```python
from build123d import *

# Parameters (mm, degrees)
SKETCH_1_R          = 17.5
EXTRUDE_1_DEPTH     = 3
CUT_EXTRUDE_1_REACH = 26.93
SKETCH_2_R          = 1.25
CUT_EXTRUDE_2_REACH = 26.93
SKETCH_3_R          = 1.25
CUT_EXTRUDE_3_REACH = 26.93
SKETCH_4_R          = 7.5
CUT_EXTRUDE_4_REACH = 26.93
FILLET_1_R          = 3
SKETCH_8_R          = 3
CUT_EXTRUDE_5_DEPTH = 2


with BuildPart() as part:
    # 草图1 → 凸台-拉伸1 (new body)
    with BuildSketch(Plane.XY):
        Circle(SKETCH_1_R)
    extrude(amount=EXTRUDE_1_DEPTH)

    # 草图2 → 切除-拉伸1 (cut, up to next)
    with BuildSketch(Plane(origin=(0, 0, 0), x_dir=(-1, 0, 0), z_dir=(0, 0, -1)), mode=Mode.PRIVATE) as cut_extrude_1_sk1:
        with Locations((-8.838834765, 8.838834765)):
            Circle(SKETCH_2_R)
    cut_extrude_1_tool1 = extrude(cut_extrude_1_sk1.sketch, amount=-CUT_EXTRUDE_1_REACH, mode=Mode.PRIVATE) & part.part
    # 草图2 → 切除-拉伸1 (cut, up to next)
    with BuildSketch(Plane(origin=(0, 0, 0), x_dir=(-1, 0, 0), z_dir=(0, 0, -1)), mode=Mode.PRIVATE) as cut_extrude_1_sk2:
        with Locations((8.838834765, 8.838834765)):
            Circle(SKETCH_2_R)
    cut_extrude_1_tool2 = extrude(cut_extrude_1_sk2.sketch, amount=-CUT_EXTRUDE_1_REACH, mode=Mode.PRIVATE) & part.part
    # 草图2 → 切除-拉伸1 (cut, up to next)
    with BuildSketch(Plane(origin=(0, 0, 0), x_dir=(-1, 0, 0), z_dir=(0, 0, -1)), mode=Mode.PRIVATE) as cut_extrude_1_sk3:
        with Locations((8.838834765, -8.838834765)):
            Circle(SKETCH_2_R)
    cut_extrude_1_tool3 = extrude(cut_extrude_1_sk3.sketch, amount=-CUT_EXTRUDE_1_REACH, mode=Mode.PRIVATE) & part.part
    # 草图2 → 切除-拉伸1 (cut, up to next)
    with BuildSketch(Plane(origin=(0, 0, 0), x_dir=(-1, 0, 0), z_dir=(0, 0, -1)), mode=Mode.PRIVATE) as cut_extrude_1_sk4:
        with Locations((-8.838834765, -8.838834765)):
            Circle(SKETCH_2_R)
    cut_extrude_1_tool4 = extrude(cut_extrude_1_sk4.sketch, amount=-CUT_EXTRUDE_1_REACH, mode=Mode.PRIVATE) & part.part
    add(cut_extrude_1_tool1.solids().sort_by_distance((8.838835, 8.838835, 0))[0], mode=Mode.SUBTRACT)
    add(cut_extrude_1_tool2.solids().sort_by_distance((-8.838835, 8.838835, 0))[0], mode=Mode.SUBTRACT)
    add(cut_extrude_1_tool3.solids().sort_by_distance((-8.838835, -8.838835, 0))[0], mode=Mode.SUBTRACT)
    add(cut_extrude_1_tool4.solids().sort_by_distance((8.838835, -8.838835, 0))[0], mode=Mode.SUBTRACT)

    # 草图3 → 切除-拉伸2 (cut, up to next)
    with BuildSketch(Plane(origin=(0, 0, 0), x_dir=(-1, 0, 0), z_dir=(0, 0, -1)), mode=Mode.PRIVATE) as cut_extrude_2_sk1:
        with Locations((0, 10.606601718)):
            Circle(SKETCH_3_R)
    cut_extrude_2_tool1 = extrude(cut_extrude_2_sk1.sketch, amount=-CUT_EXTRUDE_2_REACH, mode=Mode.PRIVATE) & part.part
    # 草图3 → 切除-拉伸2 (cut, up to next)
    with BuildSketch(Plane(origin=(0, 0, 0), x_dir=(-1, 0, 0), z_dir=(0, 0, -1)), mode=Mode.PRIVATE) as cut_extrude_2_sk2:
        with Locations((-10.606601718, 0)):
            Circle(SKETCH_3_R)
    cut_extrude_2_tool2 = extrude(cut_extrude_2_sk2.sketch, amount=-CUT_EXTRUDE_2_REACH, mode=Mode.PRIVATE) & part.part
    # 草图3 → 切除-拉伸2 (cut, up to next)
    with BuildSketch(Plane(origin=(0, 0, 0), x_dir=(-1, 0, 0), z_dir=(0, 0, -1)), mode=Mode.PRIVATE) as cut_extrude_2_sk3:
        with Locations((0, -10.606601718)):
            Circle(SKETCH_3_R)
    cut_extrude_2_tool3 = extrude(cut_extrude_2_sk3.sketch, amount=-CUT_EXTRUDE_2_REACH, mode=Mode.PRIVATE) & part.part
    # 草图3 → 切除-拉伸2 (cut, up to next)
    with BuildSketch(Plane(origin=(0, 0, 0), x_dir=(-1, 0, 0), z_dir=(0, 0, -1)), mode=Mode.PRIVATE) as cut_extrude_2_sk4:
        with Locations((10.606601718, 0)):
            Circle(SKETCH_3_R)
    cut_extrude_2_tool4 = extrude(cut_extrude_2_sk4.sketch, amount=-CUT_EXTRUDE_2_REACH, mode=Mode.PRIVATE) & part.part
    add(cut_extrude_2_tool1.solids().sort_by_distance((0, 10.606602, 0))[0], mode=Mode.SUBTRACT)
    add(cut_extrude_2_tool2.solids().sort_by_distance((10.606602, 0, 0))[0], mode=Mode.SUBTRACT)
    add(cut_extrude_2_tool3.solids().sort_by_distance((0, -10.606602, 0))[0], mode=Mode.SUBTRACT)
    add(cut_extrude_2_tool4.solids().sort_by_distance((-10.606602, 0, 0))[0], mode=Mode.SUBTRACT)

    # 草图4 → 切除-拉伸3 (cut, up to next)
    with BuildSketch(Plane(origin=(0, 0, 0), x_dir=(-1, 0, 0), z_dir=(0, 0, -1)), mode=Mode.PRIVATE) as cut_extrude_3_sk1:
        Circle(SKETCH_4_R)
    cut_extrude_3_tool1 = extrude(cut_extrude_3_sk1.sketch, amount=-CUT_EXTRUDE_3_REACH, mode=Mode.PRIVATE) & part.part
    add(cut_extrude_3_tool1.solids().sort_by_distance((0, 0, 0))[0], mode=Mode.SUBTRACT)

    # 草图7 → 切除-拉伸4 (cut, up to next)
    with BuildSketch(Plane.XY.offset(3), mode=Mode.PRIVATE) as cut_extrude_4_sk1:
        with BuildLine():
            Line((-12.374368671, 12.374368671), (12.374368671, 12.374368671))
            ThreePointArc((12.374368671, 12.374368671), (0, 17.5), (-12.374368671, 12.374368671))
        make_face()
    cut_extrude_4_tool1 = extrude(cut_extrude_4_sk1.sketch, amount=-CUT_EXTRUDE_4_REACH, mode=Mode.PRIVATE) & part.part
    # 草图7 → 切除-拉伸4 (cut, up to next)
    with BuildSketch(Plane.XY.offset(3), mode=Mode.PRIVATE) as cut_extrude_4_sk2:
        with BuildLine():
            Line((12.374368671, 12.374368671), (12.374368671, -12.374368671))
            ThreePointArc((12.374368671, -12.374368671), (16.167891819, -6.696960066), (17.5, 0))
            ThreePointArc((17.5, 0), (16.167891819, 6.696960066), (12.374368671, 12.374368671))
        make_face()
    cut_extrude_4_tool2 = extrude(cut_extrude_4_sk2.sketch, amount=-CUT_EXTRUDE_4_REACH, mode=Mode.PRIVATE) & part.part
    # 草图7 → 切除-拉伸4 (cut, up to next)
    with BuildSketch(Plane.XY.offset(3), mode=Mode.PRIVATE) as cut_extrude_4_sk3:
        with BuildLine():
            ThreePointArc((-12.374368671, -12.374368671), (0, -17.5), (12.374368671, -12.374368671))
            Line((12.374368671, -12.374368671), (-12.374368671, -12.374368671))
        make_face()
    cut_extrude_4_tool3 = extrude(cut_extrude_4_sk3.sketch, amount=-CUT_EXTRUDE_4_REACH, mode=Mode.PRIVATE) & part.part
    # 草图7 → 切除-拉伸4 (cut, up to next)
    with BuildSketch(Plane.XY.offset(3), mode=Mode.PRIVATE) as cut_extrude_4_sk4:
        with BuildLine():
            ThreePointArc((-12.374368671, 12.374368671), (-17.5, 0), (-12.374368671, -12.374368671))
            Line((-12.374368671, -12.374368671), (-12.374368671, 12.374368671))
        make_face()
    cut_extrude_4_tool4 = extrude(cut_extrude_4_sk4.sketch, amount=-CUT_EXTRUDE_4_REACH, mode=Mode.PRIVATE) & part.part
    add(cut_extrude_4_tool1.solids().sort_by_distance((0, 14.452754, 3))[0], mode=Mode.SUBTRACT)
    add(cut_extrude_4_tool2.solids().sort_by_distance((14.452754, 0, 3))[0], mode=Mode.SUBTRACT)
    add(cut_extrude_4_tool3.solids().sort_by_distance((0, -14.452754, 3))[0], mode=Mode.SUBTRACT)
    add(cut_extrude_4_tool4.solids().sort_by_distance((-14.452754, 0, 3))[0], mode=Mode.SUBTRACT)

    # 圆角1
    fillet_1_edges = [part.edges().sort_by_distance(p)[0] for p in [
        (12.374368671, 12.374368671, 1.5),
        (-12.374368671, 12.374368671, 1.5),
        (-12.374368671, -12.374368671, 1.5),
        (12.374368671, -12.374368671, 1.5),
    ]]
    fillet(fillet_1_edges, radius=FILLET_1_R)

    # 草图8 → 切除-拉伸5 (cut)
    with BuildSketch(Plane.XY.offset(3)):
        with Locations((-8.838834765, 8.838834765)):
            Circle(SKETCH_8_R)
        with Locations((8.838834765, 8.838834765)):
            Circle(SKETCH_8_R)
        with Locations((8.838834765, -8.838834765)):
            Circle(SKETCH_8_R)
        with Locations((-8.838834765, -8.838834765)):
            Circle(SKETCH_8_R)
    extrude(amount=-CUT_EXTRUDE_5_DEPTH, mode=Mode.SUBTRACT)


solid = part.part
```
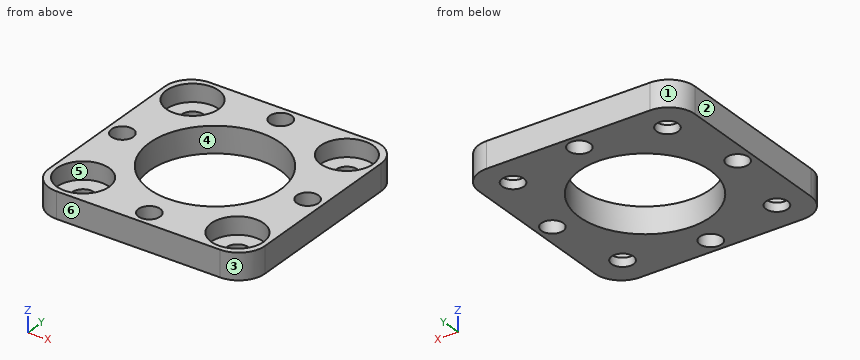
Check sheet for the modelled part. Datum: model origin and axes. Units: mm. Face numbers are marked on the shaded views. A direction names the side the tool comes from. Round coordinates to 2 decimals unless told otherwise and drop trailing zeros. Order: outer loops, then holes, each group sorted by start corner. A loop starts at its lowest first (then second) coordinate and runs counter-clockwise, first axis right, second up.
1) Scan lines: line 1 (Y direction, x = 0, z = 1.1); line 2 (Y direction, x = -6.25, z = 1.1); line 3 (X direction, y = 10, z = 1.2) (3 decimals). Record each from-to range of solid material in increasing order.
2) Tool access check on the marked faces 5 and 6. Record the directions out of +Z, -Z, +X, -X, +Y, -Y that give a thin tool (end or side, any length) a straight path to the whole face; none if there is none.
3) Go/stop test with flat-tipped pins: pin 1 Ø12 at (x, y) = (0, 0) entering from +Z; pin 2 Ø1.8 at (x, y) = (8, 9) entering from +Z. Record where each tip stops, or that it passes through.
4) Mould release check, pull along Y, two halves, no side actions. Record for the marked faces 1, 2, 3 and 4: +Y half, -Y half, draft (parallel to the pull), parting line (faces both ways), or undercut.
5) Section check A-A (y = 0). Record the boundary of the cut face in (x, z), and give its area (3 significant figures).
6) Section check B-B (x = 4.5). Record the boundary of the cut face in (y, z), and give its area (3 significant figures).
7) Section check C-C (z = 1.35). Give the number of separate pieces and of enclosed holes in the cut face, and give its area (3 significant figures).
Result:
1. line 1: y = -12.37 to -11.86, -9.36 to -7.5, 7.5 to 9.36, 11.86 to 12.37
1. line 2: y = -12.37 to -10.35, -7.32 to -4.15, 4.15 to 7.32, 10.35 to 12.37
1. line 3: x = -12.308 to -11.605, -6.073 to -1.093, 1.093 to 6.073, 11.605 to 12.308
2. face 5: +Z
2. face 6: +Z, -Z, +X, -X, -Y
3. pin 1: passes through
3. pin 2: stops at z = 1
4. face 1: +Y half
4. face 2: draft
4. face 3: -Y half
4. face 4: undercut
5. outline: (-12.37, 0) - (-11.86, 0) - (-11.86, 3) - (-12.37, 3) - close; (-9.36, 0) - (-7.5, 0) - (-7.5, 3) - (-9.36, 3) - close; (7.5, 0) - (9.36, 0) - (9.36, 3) - (7.5, 3) - close; (11.86, 0) - (12.37, 0) - (12.37, 3) - (11.86, 3) - close
5. area: 14.2 mm2
6. outline: (-12.37, 0) - (-6, 0) - (-6, 3) - (-12.37, 3) - close; (6, 0) - (12.37, 0) - (12.37, 3) - (6, 3) - close
6. area: 38.2 mm2
7. separate pieces: 1
7. enclosed holes: 9
7. area: 295 mm2
